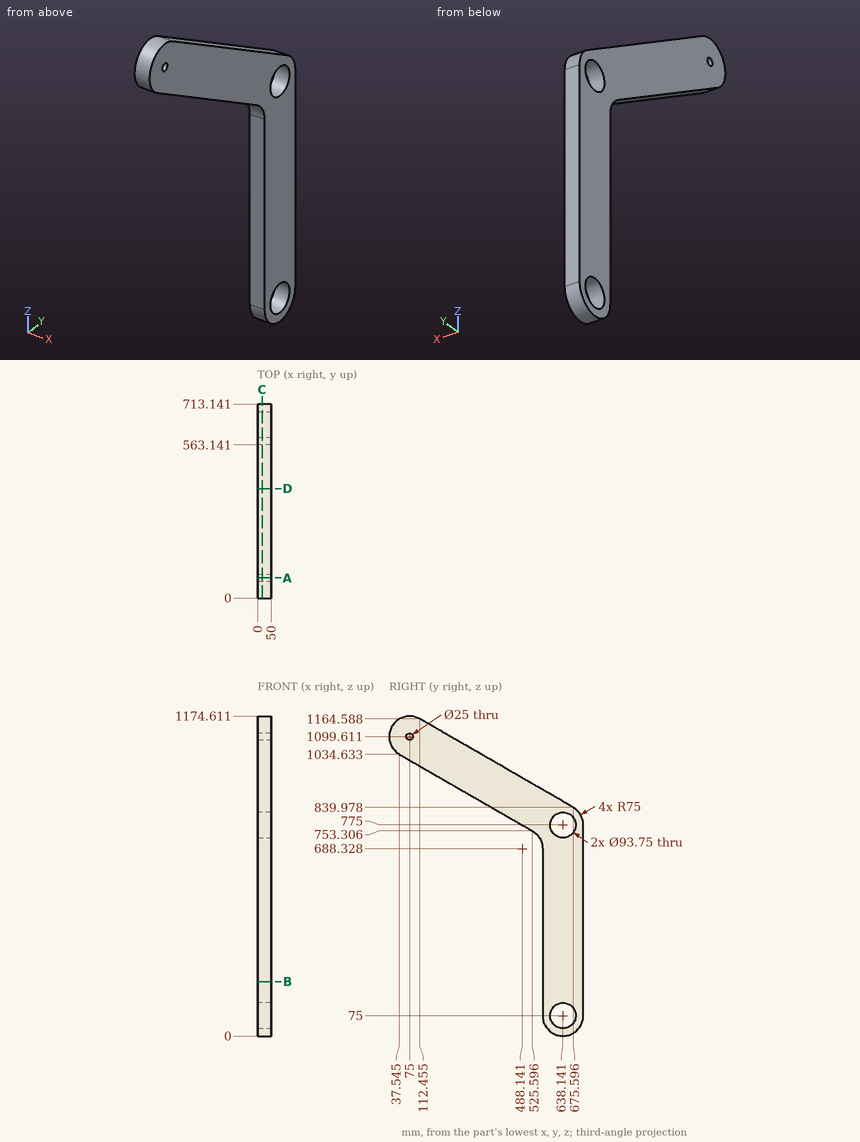
Check sheet for the drawn part. Datum: minimum x, y, z corner. Units: mm. Give positions to 0.01 mm unless a question says otherwise; leave off trailing zeros. Order: outer loops, then holes, each group sorted by start corner. A loop starts at its lowest first (then second) coordinate and runs counter-clockwise, first axis right, second up. Notation, with made-up numbers: (63, 38) -> (67, 38) arc R15 ccw to (67, 47) -> close; hole circle Ø5 at (1.25, 44.5). An arc over 180 degrees is marked (long way). Answer as CSV lines item,"result".
Q1. Depth check by flat-ended pin: pin 1 (1 mm diameter, centred on x = 33.5, y = 190.5, fed in from +Z); pin 2 (15 mm diameter, centred on x = 36.5, z = 488.5, fed in from -Y); pin 3 (8 mm diameter, centred on x = 40.5, y = 201.5, fed in from +Z) (1 decimal). Enter the tip coordinate at first touch or a pass-through.
Solutions:
pin 1,"stops at z = 1119.89"
pin 2,"stops at y = 563.14"
pin 3,"stops at z = 1115.6"
Q2. Sectioned sample at B-B on z = 199.5. Record the cut outline in (x, y).
Solutions:
outline,"(0, 563.14) -> (50, 563.14) -> (50, 713.14) -> (0, 713.14) -> close"
Q3. Sectioned sample at A-A on y = 75. Record the cut outline in (x, z), plus the area to 3 significant figures.
Solutions:
outline,"(0, 1013.04) -> (50, 1013.04) -> (50, 1087.11) -> (0, 1087.11) -> close; (0, 1112.11) -> (50, 1112.11) -> (50, 1174.61) -> (0, 1174.61) -> close"
area,"6,830 mm²"
Q4. Sectioned sample at D-D on y = 402.5. Record the cut outline in (x, z), plus the area to 3 significant figures.
Solutions:
outline,"(0, 824.26) -> (50, 824.26) -> (50, 997.4) -> (0, 997.4) -> close"
area,"8,660 mm²"
Q5. Sectioned sample at C-C on x = 17. Count the separate pieces of the cut face and the enclosed holes in it, plus the area to 3 significant figures.
Solutions:
separate pieces,"1"
enclosed holes,"3"
area,"206,000 mm²"
Q6. Scan lines: probe 1 along Y at (x, z) = (17, 75); probe 2 along Y at (x, z) = (39, 775) (1 decimal); probe 3 along Y at (x, z) = (45.5, 657.5). Record each from-to range of solid material in increasing order.
Solutions:
probe 1,"y = 563.14 to 591.27, 685.02 to 713.14"
probe 2,"y = 488 to 591.3, 685 to 713.1"
probe 3,"y = 563.14 to 713.14"
